Autodesk Inventor part; units mm, degrees
ref_plane "YZ Plane" through (0, 0, 0) normal (1, 0, 0) x (0, 1, 0)
ref_plane "XZ Plane" through (0, 0, 0) normal (0, 1, 0) x (-1, 0, 0)
ref_plane "XY Plane" through (0, 0, 0) normal (0, 0, 1) x (1, 0, 0)
sketch "Эскиз1" plane through (0, 0, 0) normal (0, 1, 0) x (-1, 0, 0)
  line L0 (0, 0) -> (16.5, 0)
  line L1 (16.5, 0) -> (16.5, -18)
  line L2 (16.5, -18) -> (0, -18)
  line L3 (0, -18) -> (0, 0)
  dimension "d0" = 16.5
  dimension "d1" = 18
extrude "Выдавливание1" add sketch "Эскиз1" along normal blind 1.5
sketch "Эскиз2" plane through (0, 1.5, 0) normal (0, 1, 0) x (1, 0, 0)
  line L0 (-16.5, 18) -> (-16.5, 0)
  line L1 (-16.5, 0) -> (0, 0) construction
  line L2 (-8.25, 0) -> (-8.25, 18) construction
  line L3 (0, 18) -> (-16.5, 18) construction
  line L4 (-15.87, 2.65) -> (-15.87, 0) construction
  line L5 (-15.87, 15.35) -> (-15.87, 18) construction
  line L6 (-15.87, 2.65) -> (-16.5, 2.65) construction
  point P0 (-15.87, 12.81)
  point P1 (-15.87, 10.27)
  point P2 (-15.87, 7.73)
  point P3 (-15.87, 5.19)
  point P4 (-0.63, 15.35)
  point P5 (-0.63, 12.81)
  point P6 (-0.63, 10.27)
  point P7 (-0.63, 7.73)
  point P8 (-0.63, 5.19)
  point P9 (-0.63, 2.65)
  dimension "d6" = 2.54
  dimension "d11" = 15.24
hole "Отверстие1" at (-15.87, 1.5, -15.35) at (-15.87, 1.5, -12.81) at (-15.87, 1.5, -10.27) at (-15.87, 1.5, -7.73) at (-15.87, 1.5, -5.19) at (-15.87, 1.5, -2.65) at (-0.63, 1.5, -2.65) at (-0.63, 1.5, -5.19) at (-0.63, 1.5, -7.73) at (-0.63, 1.5, -10.27) at (-0.63, 1.5, -12.81) at (-0.63, 1.5, -15.35) direction (0, -1, 0) diameter 0.8 end through all
properties part number "Драйвер моторов DRV8833"
For this review, take the finished solid that the model builds, in its own axes (mm). Coordinates: 2 decimals unless noted, no trailing zeros. Order: outer loops, then holes, each group sorted by start corner. A loop starts at its lowest first (then second) coordinate and runs counter-clockwise, first axis right, second up. Notation, with made-up numbers: (46.5, 13.25) - (50.5, 13.25) arc R24 ccw to (50.5, 41.25) - close; hole circle Ø2 at (28.5, -34). An arc over 180 degrees is marked (long way). Answer as CSV lines item,"result". Start each with the question number.
1) Add section B-B (z = -5.19). State the section outline as (x, y) points.
2) To check wall thickness, follow line 1 along X through (y, z) = (0.6, -5.19); line 2 along X through (y, z) = (0.35, -5.5). State the ranges of each line that lie inside material, in increasing order. Write a range as [from, to].
3) Add section A-A (y = 0.25). Count the separate pieces of the cut face and the enclosed holes in it, then the cut area to 3 significant figures.
4) Add section C-C (x = -0.63). State the section outline as (y, z) points, then the cut area to 3 significant figures.
5) Draft analysis for pull direction Z (two halves, no side actions). For faces 1 (the cylindrical face through (-15.515, 0.74, -5.005)), 2 (the flat face through (-8, 0, -9)), 3 (the flat face through (-8, 1, 0)), state which applies: +Z half, -Z half, draft (parallel to the pull), parting line (faces both ways), or undercut.
Result:
1,outline,"(-16.5, 0) - (-16.27, 0) - (-16.27, 1.5) - (-16.5, 1.5) - close; (-15.47, 0) - (-1.03, 0) - (-1.03, 1.5) - (-15.47, 1.5) - close; (-0.23, 0) - (0, 0) - (0, 1.5) - (-0.23, 1.5) - close"
2,line 1,"[-16.5, -16.27], [-15.47, -1.03], [-0.23, 0]"
2,line 2,"[-16.5, -16.12], [-15.62, -0.88], [-0.38, 0]"
3,separate pieces,"1"
3,enclosed holes,"12"
3,area,"291 mm^2"
4,outline,"(0, -18) - (1.5, -18) - (1.5, -15.75) - (0, -15.75) - close; (0, -14.95) - (1.5, -14.95) - (1.5, -13.21) - (0, -13.21) - close; (0, -12.41) - (1.5, -12.41) - (1.5, -10.67) - (0, -10.67) - close; (0, -9.87) - (1.5, -9.87) - (1.5, -8.13) - (0, -8.13) - close; (0, -7.33) - (1.5, -7.33) - (1.5, -5.59) - (0, -5.59) - close; (0, -4.79) - (1.5, -4.79) - (1.5, -3.05) - (0, -3.05) - close; (0, -2.25) - (1.5, -2.25) - (1.5, 0) - (0, 0) - close"
4,area,"19.8 mm^2"
5,face 1,"undercut"
5,face 2,"draft"
5,face 3,"+Z half"
